Autodesk Inventor part; units mm, degrees
ref_plane "Work Plane3" through (-14.15, 0, 1.3711) normal (1, 0, 0) x (0, 0, -1)
ref_plane "Work Plane4" through (0, 7.5, 0) normal (0, -1, 0) x (1, 0, 0)
ref_plane "YZ Plane" through (0, 0, 0) normal (1, 0, 0) x (0, 1, 0)
sketch "Sketch1" plane through (0, 0, 0) normal (0, 1, 0) x (-1, 0, 0)
  arc A0 (2.15, 1.3711) -> (2.15, -1.3711) centre (0, 0) ccw
  line L0 (2.15, 1.3711) -> (2.15, -1.3711)
  dimension "d1" = 4.7
  dimension "d92" = 2.55
sketch "Sketch2" plane through (0, 0, 0) normal (1, 0, 0) x (0, 1, 0)
  line L0 (0, 0) -> (15, 0)
  line L1 (15, 0) -> (15, -14)
  line L2 (0, 0) -> (0, -14)
  line L3 (5, -10) -> (15, -17.0021)
  line L4 (15, -14) -> (15, -17.0021)
  line L5 (7.5, 0) -> (7.5, -2.5713) construction
  line L6 (10, -10) -> (0, -17.0021)
  line L7 (0, -14) -> (0, -17.0021)
  point P0 (7.5, -11.7505)
  dimension "d4" = 15
  dimension "d5" = 14
  dimension "d6" = 14
  dimension "d93" = 10
  dimension "d102" = 55
  dimension "d103" = 10
revolve "Revolution1" add sketch "Sketch2" angle 360 about axis through (0, 0, 0) along (0, 1, 0)
extrude "Extrusion1" cut sketch "Sketch1" along normal through all
chamfer "Chamfer1" distance 1.2 angle 45 2 edges at (0, 15, 17.0021) (0, 0, 17.0021)
ref_plane "Work Plane3" through (-14.15, 0, 1.3711) normal (1, 0, 0) x (0, 0, -1)
ref_plane "Work Plane4" through (0, 7.5, 0) normal (0, -1, 0) x (1, 0, 0)
fillet "Fillet1" radius 2 1 edges at (0, 7.5, 11.7505)
chamfer "Chamfer2" distance 1 angle 45 2 edges at (-2.15, 0, 0) (2.55, 0, 0)
hole "Hole4" at (0, 0, 0) direction (0, 1, 0) diameter 6.5 depth 5.3
chamfer "Chamfer3" distance 0.2 angle 45 3 edges at (-2.15, 5.3, 0) (2.55, 5.3, 0) (0, 5.3, 3.25)
equation "\"d6\" = d5"
properties part number "Stepper Pulley V12_3DPrint"
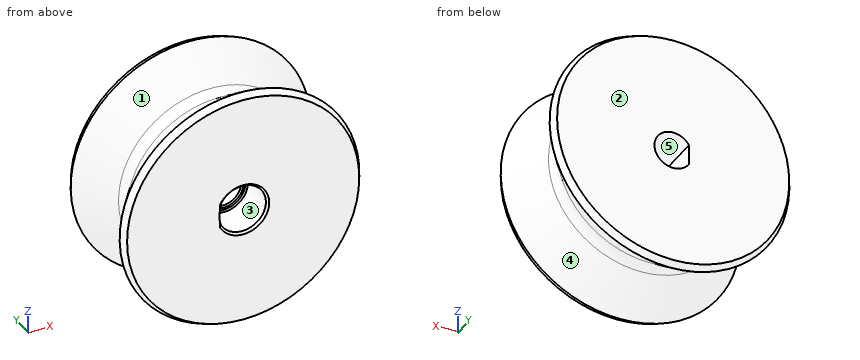
Read the model definition and answer for the solid it produces. Units are mm, in the model's axes. Face numbers are marked on the shaded views. A direction names the side the tool comes from. Give positions to 0.01 mm unless a question says otherwise; leave off trailing zeros. Order: outer loops, then holes, each group sorted by start corner. A loop starts at its lowest first (then second) coordinate and runs counter-clockwise, first axis right, second up.
(1) Straight lines are drawn through the part: L1, parallel to Y at x = -8, z = -9.5; L2, parallel to Y at x = -7, z = 12; L3, parallel to Z at x = 2, y = 11. For each, find the intervals that lie inside material, in ascending order.
(2) For the marked faces 4 and 5, determine the directions among +Z, -Z, +X, -X, +Y, -Y from which every point of the face is accessible in a straight line to the end or side of a thin tool.
(3) Find section A-A (y = 3). Give the vertices of the cut face in (x, z), plus the area to 3 significant figures.
(4) For a pull along Z with two mould halves and no side action, classify the marked faces 1, 2 and 3 as released by +Z, released by -Z, zero draft, split by the parting line, or undercut.
(5) Given pin 1 (2 mm diameter, centred on x = 4.5, y = 9, fed in from -Z); pin 2 (2 mm diameter, centred on y = 11.5, z = 0.5, fed in from +X); pin 3 (3 mm diameter, centred on x = 1, z = -0.5, fed in from -Y), each flat-ended and moving along its own axis, determine where each tip first touches the part or whether it passes through.
Result sheet:
1. L1: y = 0 to 6.57, 8.43 to 15
1. L2: y = 0 to 4.44, 10.56 to 15
1. L3: z = -14.06 to -1.58, 1.58 to 14.06
2. face 4: none
2. face 5: +Y, -Y
3. outline: circle Ø29.8 at (0, 0); hole circle Ø6.5 at (0, 0)
3. area: 664 mm2
4. face 1: split by the parting line
4. face 2: zero draft
4. face 3: undercut
5. pin 1: stops at z = -12.8
5. pin 2: stops at x = 15.24
5. pin 3: stops at y = 5.43
